Read the model definition and answer for the solid it produces. Units are mm, in the model's axes. A direction names the side the tool comes from. Coordinates: 2 decimals unless noted, no trailing zeros. Loops run counter-clockwise (first coordinate to the right, second up) from the corner with the lowest first, then second, coordinate; pieces in that order, holes last. Notation, with made-up numbers: M -16,87.5 L 24,87.5 A19 ccw 24,92.5 Z; hole C -6.75,54.5 d7. An arc over 180 degrees is marked long. One line per item, written item: value. Start each with the question number.
1. Consider probe 1 along Y at (x, z) = (8.95, 11.25); probe 2 along Z at (x, y) = (2.5, 19.5); probe 3 along Y at (x, z) = (4, 11). Determine where each line is inside the solid, lowest interval first.
2. The part is cut by section B-B (y = 0). Write down the section's boundary in (x, z), then the cut area to 3 significant figures.
3. The part is cut by section D-D (z = -11.25). State how many separate pieces and enclosed holes the cut face has, then the cut area to 3 significant figures.
4. Flat-ended cylindrical pins translate along their axes: pin 1 (2 mm diameter, centred on x = -29.5, y = 7.5, fed in from +Z); pin 2 (1 mm diameter, centred on x = -11.5, z = 8, fed in from +Y); pin 3 (7.5 mm diameter, centred on y = -19, z = 10.5, fed in from +X); pin 4 (9 mm diameter, centred on y = 0, z = 0, fed in from -X). Find the tip coordinate at first contact, or state that the pin passes through.
5. The part is cut by section A-A (z = 0). Write down the section's boundary in (x, y).
6. Determine the mould class of faces 5 (the face through (-32, 0, 13)), 6 (the face through (8.35, 20.345, 0.738)) for opening direction X: +X half, -X half, draft (parallel to the pull), parting line (faces both ways), or undercut.
7. The part is cut by section C-C (y = -18.5). Write down the section's boundary in (x, z).
8. For faces 1 (the face through (-0.8, -5, -16)), 2 (the face through (-17, 0, 16)), 3 (the face through (-19.958, -0.747, -16.984)), 4 (the face through (9.042, -24.123, -10.22)), determine the directions among +Z, -Z, +X, -X, +Y, -Y from which every point of the face is accessible in a straight line to the end or side of a thin tool.
```python
from build123d import *

# Parameters (mm, degrees)
CUT_EXTRUDE1_DEPTH                 = 58.28874235
CHAMFER1_SIZE                      = 0.34
SOCKET_HEAD_CAP_SCREW1_D           = 6
SOCKET_HEAD_CAP_SCREW1_CBORE_D     = 9.5
SOCKET_HEAD_CAP_SCREW1_CBORE_DEPTH = 6
CUT_EXTRUDE2_DEPTH                 = 35
BOSS_EXTRUDE1_DEPTH                = 5
SKETCH7_R                          = 1.5
BOSS_EXTRUDE2_DEPTH                = 1
REVOLVE3_ANGLE                     = 90
REVOLVE4_ANGLE                     = 90
TAP1_START                         = 4.7999999
TAP1_OUTLINE_R                     = 2.4585
TAP1_DEPTH                         = 7.2000001


# Read off the part's stored shape, not the designer's step: Tap1
with BuildPart() as part:
    # Sketch1 → Revolve1 (revolve)
    with BuildSketch(Plane.XY, mode=Mode.PRIVATE) as revolve1_sk:
        Polygon((0, 29), (12, 29), (12, 7.5), (-40, 7.5), (-40, 17), (-0.8, 17), (-0.8, 16.32), (0, 16.32), align=None)
    revolve(revolve1_sk.sketch.rotate(Axis((-40, 0, 0), (1, 0, 0)), 90), axis=Axis((-40, 0, 0), (1, 0, 0)))

    # Sketch2 → Cut-Extrude1 (cut, through all)
    with BuildSketch(Plane(origin=(0, 0, 0), x_dir=(0, 0, -1), z_dir=(1, 0, 0))):
        with BuildLine():
            Line((14.696938457, 25), (-14.696938457, 25))
            ThreePointArc((-14.696938457, 25), (0, 29), (14.696938457, 25))
        make_face()
        with BuildLine():
            Line((17, 23.494680249), (17, -23.494680249))
            ThreePointArc((17, -23.494680249), (29, 0), (17, 23.494680249))
        make_face()
        with BuildLine():
            Line((14.696938457, -25), (-14.696938457, -25))
            ThreePointArc((-14.696938457, -25), (0, -29), (14.696938457, -25))
        make_face()
        with BuildLine():
            Line((-17, -23.494680249), (-17, 23.494680249))
            ThreePointArc((-17, 23.494680249), (-29, 0), (-17, -23.494680249))
        make_face()
    extrude(amount=CUT_EXTRUDE1_DEPTH, mode=Mode.SUBTRACT)

    # Chamfer1
    chamfer1_edges = [part.edges().sort_by_distance(p)[0] for p in [
        (-40, 0, -17),
    ]]
    chamfer(chamfer1_edges, length=CHAMFER1_SIZE)

    # Socket Head Cap Screw1 (through all)
    with Locations(Plane(origin=(12, 0, 0), x_dir=(0, 0, -1), z_dir=(1, 0, 0))):
        with Locations((-11.25, 19.485571585), (11.25, -19.485571585), (-11.25, -19.485571585), (11.25, 19.485571585)):
            CounterBoreHole(SOCKET_HEAD_CAP_SCREW1_D / 2, SOCKET_HEAD_CAP_SCREW1_CBORE_D / 2, SOCKET_HEAD_CAP_SCREW1_CBORE_DEPTH)

    # Sketch5 → Cut-Extrude2 (cut)
    with BuildSketch(Plane(origin=(0, 0, 0), x_dir=(0, 0, -1), z_dir=(1, 0, 0))):
        with BuildLine():
            Line((-11, -12.961481397), (-11, 12.961481397))
            ThreePointArc((-11, 12.961481397), (-17, 0), (-11, -12.961481397))
        make_face()
    extrude(amount=-CUT_EXTRUDE2_DEPTH, mode=Mode.SUBTRACT)

    # Sketch6 → Boss-Extrude1 (add)
    with BuildSketch(Plane(origin=(0, 0, 11), x_dir=(-1, 0, 0), z_dir=(0, 0, -1))):
        with BuildLine():
            Line((6, 4), (28, 4))
            ThreePointArc((28, 4), (32, 0), (28, -4))
            Line((28, -4), (6, -4))
            ThreePointArc((6, -4), (2, 0), (6, 4))
        make_face()
    extrude(amount=-BOSS_EXTRUDE1_DEPTH)

    # Sketch7 → Boss-Extrude2 (add)
    with BuildSketch(Plane(origin=(0, 0, 11), x_dir=(-1, 0, 0), z_dir=(0, 0, -1))):
        with Locations(Location((27.571413315, -8.870469014, 0), (0, 0, 180))):
            Circle(SKETCH7_R)
        with Locations(Location((6.428586685, 8.870469014, 0), (0, 0, 180))):
            Circle(SKETCH7_R)
    extrude(amount=-BOSS_EXTRUDE2_DEPTH)

    # Sketch8 → Revolve2 (revolve)
    with BuildSketch(Plane.XY.offset(12)):
        Polygon((-27.571413315, -8.870469014), (-6.428586685, 8.870469014), (-7.392768099, 10.019535678), (-28.53559473, -7.721402349), align=None)
    revolve(axis=Axis((-27.571413315, -8.870469014, 12), (0.7660444431189788, 0.6427876096865385, 0)))

    # Sketch9 → Revolve3 (revolve)
    with BuildSketch(Plane.XY.offset(12)):
        with BuildLine():
            Line((-26.607231901, -10.019535678), (-28.53559473, -7.721402349))
            ThreePointArc((-28.53559473, -7.721402349), (-28.72047998, -9.834650428), (-26.607231901, -10.019535678))
        make_face()
    revolve(axis=Axis((-26.607231901, -10.019535678, 12), (-0.6427876096865375, 0.7660444431189796, 0)), revolution_arc=REVOLVE3_ANGLE)

    # Sketch10 → Revolve4 (revolve)
    with BuildSketch(Plane.XY.offset(12)):
        with BuildLine():
            Line((-7.392768099, 10.019535678), (-5.46440527, 7.721402349))
            ThreePointArc((-5.46440527, 7.721402349), (-5.27952002, 9.834650428), (-7.392768099, 10.019535678))
        make_face()
    revolve(axis=Axis((-7.392768099, 10.019535678, 12), (0.6427876096865389, -0.7660444431189785, 0)), revolution_arc=REVOLVE4_ANGLE)

    # Sketch11 → Cut-Revolve1 (revolve, cut)
    with BuildSketch(Plane.XY, mode=Mode.PRIVATE) as cut_revolve1_sk:
        with BuildLine():
            Line((2.3, 0), (4.8, 0))
            Line((4.8, 0), (4.8, 20.4585))
            ThreePointArc((4.8, 20.4585), (3.032233047, 19.726266953), (2.3, 17.9585))
            Line((2.3, 17.9585), (2.3, 0))
        make_face()
    revolve(cut_revolve1_sk.sketch.rotate(Axis((4.8, 0, 0), (0, 1, 0)), 270), axis=Axis((4.8, 0, 0), (0, 1, 0)), mode=Mode.SUBTRACT)

    # Tap1 outline → Tap1 (cut)
    with BuildSketch(Plane.YZ.offset(TAP1_START)):
        with Locations((18, 0)):
            Circle(TAP1_OUTLINE_R)
    extrude(amount=TAP1_DEPTH, mode=Mode.SUBTRACT)


solid = part.part
```
Answer block:
1. probe 1: y = -25 to -24.24, -14.74 to 14.74, 24.24 to 25
1. probe 2: z = -17 to -14.25, -8.25 to 8.25, 14.25 to 17
1. probe 3: y = -25 to -22.48, -16.5 to 16.5, 22.48 to 25
2. outline: M -40,-16.66 L -39.66,-17 L -0.8,-17 L -0.8,-16.32 L 0,-16.32 L 0,-17 L 12,-17 L 12,-7.5 L -40,-7.5 Z; M -40,7.5 L 12,7.5 L 12,17 L 0,17 L 0,11 L -2,11 L -2,16 L -32,16 L -32,11 L -35,11 L -35,17 L -39.66,17 L -40,16.66 Z
2. area: 927 mm2
3. separate pieces: 3
3. enclosed holes: 0
3. area: 1,430 mm2
4. pin 1: stops at z = 11
4. pin 2: stops at y = 15.26
4. pin 3: stops at x = 6
4. pin 4: passes through
5. outline: M -40,-16.66 L -39.66,-17 L -0.8,-17 L -0.8,-16.32 L 0,-16.32 L 0,-25 L 12,-25 L 12,-7.5 L -40,-7.5 Z; M -40,7.5 L 2.3,7.5 L 2.3,17.96 A2.5 cw 4.8,20.46 L 12,20.46 L 12,25 L 0,25 L 0,16.32 L -0.8,16.32 L -0.8,17 L -39.66,17 L -40,16.66 Z; M 7.3,7.5 L 12,7.5 L 12,15.54 L 7.3,15.54 Z
6. face 5: undercut
6. face 6: draft
7. outline: M 0,-17 L 12,-17 L 12,-15.9 L 6,-15.9 L 6,-14.08 L 0,-14.08 Z; M 0,-8.42 L 6,-8.42 L 6,-6.6 L 12,-6.6 L 12,6.6 L 6,6.6 L 6,8.42 L 0,8.42 Z; M 0,14.08 L 6,14.08 L 6,15.9 L 12,15.9 L 12,17 L 0,17 Z
8. face 1: none
8. face 2: +Z, +Y, -Y
8. face 3: -X
8. face 4: +X
